Geometry check sheet. Reference: the model listing, model coordinates, mm. A direction names the side the tool comes from. Coordinates: 2 decimals unless noted, no trailing zeros. Answer in a Markdown table with one row per item. Add a question column.
Q1. Gauge pin test, flat ends, axial feed: P1, Ø1.8, axis at x = 4, z = 5, coming from the -Y side; P2, Ø1.1, axis at x = -3, z = 4, coming from the +Y side; P3, Ø1.6, axis at x = -16, z = 4, coming from the -Y side; P4, Ø10, axis at x = -22.5, y = -21, coming from the -Z side. Record the tip position at first contact, or that the pin passes through.
Q2. Release check for a two-part mould opening along X. For faces 1 (the face through (8.354, 23.762, 4.93)), 2 (the face through (16.888, -7.765, 5.316)), 3 (the face through (-19.36, 12.69, 4.93)) record: pulls with the +X half, pulls with the -X half, needs draft (parallel to the pull), parting line crosses it, or undercut.
Q3. Thickness scan on line 1 (X direction, y = -18, z = 1.75); line 2 (X direction, y = -20, z = 4.25); line 3 (Z direction, x = -3, y = 12.5). Record the ranges inside material, lowest first.
Q4. Tool access check on faces 4 (the face through (-25.164, -13.739, 4.93)), 5 (the face through (33.026, -33.2, 5.316)), 6 (the face through (-0.865, -18.049, 4.93)), 7 (the face through (15, 21.314, 5)). Record the directions out of +Z, -Z, +X, -X, +Y, -Y that give a thin tool (end or side, any length) a straight path to the whole face; none if there is none.
```python
from build123d import *

# Parameters (mm, degrees)
F1_DEPTH = 10
F2_T     = -0.762
F3_R     = 12.7550536122
F4_DEPTH = 25.4


with BuildPart() as f1:
    # F0 (on Top) → F1 (new body)
    with BuildSketch(Plane.XY):
        Polygon((-7.8007113189, 25.4050213844), (-14.7581025958, 20.5559302121), (-13.5356634855, 15.0533653796), (-15.0557206944, 13.5333081707), (-18.1923042983, 13.5333081707), (-20.5559276198, 11.8295696557), (-21.2681274861, 8.3783324808), (-20.012428984, 6.527827587), (-17.7791882306, 5.4171900265), (-18.1923042983, 3.4152779263), (-21.5501468629, 0), (-24.9349009246, 0), (-26.1455569416, -1.0574074695), (-26.1455569416, -5.1203737967), (-25.6145708263, -8.7974648923), (-24.9349009246, -11.7783686146), (-25.3995768726, -15.7559095406), (-24.9349009246, -16.142109525), (-23.0465140194, -16.8757408121), (-21.7977536025, -16.142109525), (-20.9150481969, -16.8757408121), (-18.1111115962, -19.8680274189), (-18.4382367879, -21.0997294635), (-19.7853650898, -21.7411002789), (-23.4853252769, -23.4957698894), (-25.3995768726, -24.8154569417), (-29.0218316621, -27.0394197407), (-30.6820981205, -29.0370528883), (-31.2679782274, -30.5143610979), (-30.6820981205, -31.0012958944), (-28.7057235837, -31.6250957549), (-25.3995768726, -31.0012958944), (-19.7853650898, -29.8160724342), (-17.3616977744, -29.0370528883), (-16.1116474631, -27.5329919434), (-12.7562444109, -23.4957698894), (-11.2979090287, -21.7411002789), (-7.2542270645, -16.8757408121), (-5.7355757302, -16.8757408121), (-3.5900974181, -18.6588838696), (-1.705969451, -18.6588838696), (0, -17.422426492), (1.1230455963, -14.8166298422), (2.4098805152, -13.2683096454), (4.6730381437, -13.2683096454), (8.788285777, -16.688561067), (14.146274887, -19.8680274189), (19.4753222167, -24.8154569417), (29.3999388814, -35.9310284257), (31.0319885612, -37.7653092146), (32.639272511, -38.2234193385), (33.4090031683, -37.7653092146), (34.4607569277, -36.5162938833), (34.4607569277, -35.1515486836), (33.0238379538, -30.7261310518), (28.2081253827, -23.798527196), (25.8020885247, -20.3280491786), (23.8092746586, -18.7650527805), (19.688764587, -16.7849324644), (16.8812572956, -11.2681994215), (18.4691958129, -4.2106937617), (19.228663871, 0), (19.228663871, 4.3211282282), (19.688764587, 4.9077547155), (19.688764587, 10.1767061278), (19.688764587, 14.4955459982), (19.688764587, 17.2170065343), (19.228663871, 19.5308034597), (17.8511645645, 20.611198619), (15.6399458647, 21.313789199), (13.8063501083, 21.313789199), (13.1918145344, 21.7957794666), (9.7170434892, 23.2172757387), (6.9530224428, 24.3228841573), (3.3282164725, 27.1658785641), (0, 28.019279857), (-4.2789963759, 27.1658785641), align=None)
    extrude(amount=F1_DEPTH)

    # F2
    f2_openings = [f1.faces().sort_by_distance(p)[0] for p in [
        (-0.450246, -1.925405, 10),
    ]]
    offset(amount=F2_T, openings=f2_openings, kind=Kind.INTERSECTION)

    # F3 (on face) → F4 (cut)
    with BuildSketch(Plane(origin=(0, 0, 0), x_dir=(1, 0, 0), z_dir=(0, 0, -1))):
        Circle(F3_R)
    extrude(amount=-F4_DEPTH, mode=Mode.SUBTRACT)


solid = f1.part
```
Calculated:
| question | item | result |
|---|---|---|
| 1 | P1 | stops at y = -13.46 |
| 1 | P2 | stops at y = 27.53 |
| 1 | P3 | stops at y = -28.36 |
| 1 | P4 | stops at z = 0 |
| 2 | face 1 | pulls with the +X half |
| 2 | face 2 | undercut |
| 2 | face 3 | pulls with the -X half |
| 3 | line 1 | x = -19.86 to -18.82, -9.18 to -8.19, -4.38 to -0.8, 11 to 12.49, 20.46 to 22.22 |
| 3 | line 2 | x = -18.15 to -17.36, -10.84 to -9.85, 14.29 to 15.41, 24.15 to 25.38 |
| 3 | line 3 | z = 0 to 0.76 |
| 4 | face 4 | +Z, -Z, -X |
| 4 | face 5 | +Z |
| 4 | face 6 | +Z, -Z, -Y |
| 4 | face 7 | +Z, -Z, +X, +Y |
